Design review of the part built by this model. Coordinates are the model's own, in mm. Round coordinates to 2 decimals unless told otherwise and drop trailing zeros. Order: outer loops, then holes, each group sorted by start corner. A loop starts at its lowest first (then second) coordinate and runs counter-clockwise, first axis right, second up. Notation, with made-up numbers: M 66.25,-26.5 L 92.25,-26.5 A16 cw 92.25,-18.5 Z; hole C 18,77 d9. An arc over 180 degrees is marked long. Use a Markdown table: item, result. Add a question column.
(1) To check wall thickness, follow probe 1 along Y at (x, z) = (1.5, 19.5); probe 2 along Y at (x, z) = (9.75, 30.5); probe 3 along Z at (x, y) = (3.25, 58). State the ranges of each line that lie inside material, in increasing order. Write a range as from..to.
(2) Take a section at A-A (x = 4.25). Write out the cut boundary in (y, z).
(3) Take a section at C-C (y = 45.5). Write out the cut boundary in (x, z).
(4) Take a section at B-B (z = 19). Write out the cut boundary in (x, y), then the cut area to 3 significant figures.
(5) The part is to be moulded in two halves that separate along Z. For faces 1 (the face through (7, -7, 51)), 2 (the face through (10, -5, 1)), say which applies: released by +Z, released by -Z, zero draft, split by the parting line, or undercut.
```python
from build123d import *

# Parameters (mm, degrees)
F0_W     = 720
F0_H     = 200
F1_DEPTH = 10
F3_DEPTH = 25
F5_DEPTH = 7


with BuildPart() as f1:
    # F0 (on Right) → F1 (new body)
    with BuildSketch(Plane.YZ):
        Rectangle(F0_W, F0_H)
    extrude(amount=F1_DEPTH)

    # F2 (on face) → F3 (cut)
    with BuildSketch(Plane.YZ.offset(10)):
        Polygon((-70, 5), (0, 5), (70, 5), (70, 50), (-70, 50), align=None)
    extrude(amount=-F3_DEPTH, mode=Mode.SUBTRACT)

    # F4 (on face) → F5 (cut)
    with BuildSketch(Plane(origin=(0, 0, 0), x_dir=(0, -1, 0), z_dir=(-1, 0, 0))):
        Polygon((-100, 5), (0, 5), (100, 5), (100, 52), (-100, 52), align=None)
    extrude(amount=-F5_DEPTH, mode=Mode.SUBTRACT)


solid = f1.part
```
Verdict:
| question | item | result |
|---|---|---|
| 1 | probe 1 | y = -360..-100, 100..360 |
| 1 | probe 2 | y = -360..-70, 70..360 |
| 1 | probe 3 | z = -100..5, 52..100 |
| 2 | outline | M -360,-100 L 360,-100 L 360,100 L -360,100 Z; hole M -100,5 L 100,5 L 100,52 L -100,52 Z |
| 3 | outline | M 0,-100 L 10,-100 L 10,5 L 0,5 Z; M 0,52 L 7,52 L 7,50 L 10,50 L 10,100 L 0,100 Z |
| 4 | outline | M 0,-360 L 10,-360 L 10,-70 L 7,-70 L 7,-100 L 0,-100 Z; M 0,100 L 7,100 L 7,70 L 10,70 L 10,360 L 0,360 Z |
| 4 | area | 5,380 mm^2 |
| 5 | face 1 | undercut |
| 5 | face 2 | zero draft |
